Autodesk Inventor part; units mm, degrees
ref_plane "YZ Plane" through (0, 0, 0) normal (1, 0, 0) x (0, 1, 0)
ref_plane "XZ Plane" through (0, 0, 0) normal (0, 1, 0) x (-1, 0, 0)
ref_plane "XY Plane" through (0, 0, 0) normal (0, 0, 1) x (1, 0, 0)
sketch "Sketch1" plane through (0, 0, 0) normal (0, 0, 1) x (1, 0, 0)
  line L0 (-12.1708, 16.0073) -> (13.2292, 16.0073)
  line L1 (13.2292, 16.0073) -> (13.2292, -34.7927)
  line L2 (13.2292, -34.7927) -> (-12.1708, -34.7927)
  line L3 (-12.1708, -34.7927) -> (-12.1708, 16.0073)
  line L4 (11.9592, 14.7373) -> (-10.9008, 14.7373)
  line L5 (-10.9008, 14.7373) -> (-10.9008, -33.5227)
  line L6 (-10.9008, -33.5227) -> (11.9592, -33.5227)
  line L7 (11.9592, -33.5227) -> (11.9592, 14.7373)
  point P0 (0, 0)
  dimension "d0" = 25.4
  dimension "d1" = 50.8
  dimension "d2" = 1.27
extrude "Extrusion1" add sketch "Sketch1" along normal blind 381
sketch "Sketch2" plane through (-12.1708, 16.0073, 0) normal (0, 1, 0) x (1, 0, 0)
  circle A0 centre (12.7, -12.7) radius 1.7272
  line L0 (25.4, 0) -> (0, 0)
  line L1 (0, 0) -> (0, -381)
  point P0 (12.1708, 0)
  dimension "d5" = 3.4544
  dimension "d6" = 12.7
  dimension "d7" = 12.7
extrude "Extrusion2" cut sketch "Sketch2" against normal through all
pattern_linear "Rectangular Pattern1" count 38 spacing 25.4 along (0, 0, 1) of "Extrusion2"
equation "\"d3\" = d13"
equation "\"d10\" = d14"
equation "\"d13\" = 381"
equation "\"d14\" = d13"
properties part number "VersaFrame (PerimeterPieceB)"
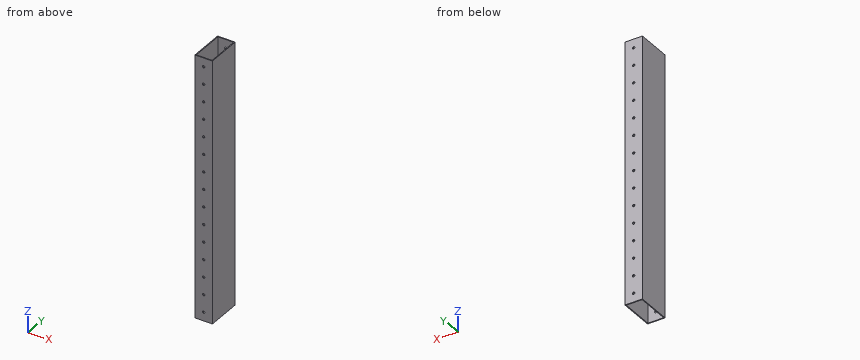
Verification items for the finished model (mm, model axes). Give positions to 0.01 mm unless a question says otherwise; leave off trailing zeros. Loops run counter-clockwise (first coordinate to the right, second up) from the corner with the lowest first, then second, coordinate; pieces in that order, holes last.
1) Sectioned sample at B-B, the plane y = -4. Enter the section's corners in (x, z), then the cut area to 3 significant figures.
2) Thickness scan on line 1 along Y through (x, z) = (5.25, 200); line 2 along X through (y, z) = (-15.5, 187.5); line 3 along X through (y, z) = (-34.25, 12.7). Record the ranges inside material, lowest first.
3) Depth check by flat-ended pin: pin 1 Ø3 at (x, z) = (0.53, 292.1) entering from -Y. Enter the tip coordinate at first touch or a pass-through.
4) Sectioned sample at A-A, the plane z = 122. Enter the section's corners in (x, y).
Answers:
1. outline: (-12.17, 0) - (-10.9, 0) - (-10.9, 381) - (-12.17, 381) - close; (11.96, 0) - (13.23, 0) - (13.23, 381) - (11.96, 381) - close
1. area: 968 mm2
2. line 1: y = -34.79 to -33.52, 14.74 to 16.01
2. line 2: x = -12.17 to -10.9, 11.96 to 13.23
2. line 3: x = -12.17 to -1.2, 2.26 to 13.23
3. pin 1: passes through
4. outline: (-12.17, -34.79) - (13.23, -34.79) - (13.23, 16.01) - (-12.17, 16.01) - close; hole (-10.9, -33.52) - (11.96, -33.52) - (11.96, 14.74) - (-10.9, 14.74) - close
